Autodesk Inventor part; units mm, degrees
ref_plane "YZ Plane" through (0, 0, 0) normal (1, 0, 0) x (0, 1, 0)
ref_plane "XZ Plane" through (0, 0, 0) normal (0, 1, 0) x (-1, 0, 0)
ref_plane "XY Plane" through (0, 0, 0) normal (0, 0, 1) x (1, 0, 0)
sketch "Sketch1" plane through (0, 0, 0) normal (0, 0, 1) x (1, 0, 0)
  arc A0 (251, 0) -> (0, 251) centre (0, 0) ccw
  arc A1 (0, 355) -> (355, 0) centre (0, 0) ccw construction
  circle A2 centre (0, 0) radius 320 construction
  line L0 (0, 0) -> (0, 251) construction
  line L1 (0, 0) -> (251, 0) construction
  arc A3 (355, 0) -> (0, 355) centre (0, 0) ccw
  line L2 (0, 251) -> (0, 355)
  arc A4 (0, 251) -> (251, 0) centre (0, 0) ccw construction
  line L3 (251, 0) -> (355, 0)
  dimension "d0" = 502
  dimension "d1" = 710
  dimension "d2" = 640
extrude "Plate1" add sketch "Sketch1" against normal blind 4
sketch "Sketch3" plane through (0, 0, 0) normal (0, 0, 1) x (1, 0, 0)
  circle A0 centre (0, 0) radius 320 construction
  line L0 (0, 0) -> (0, 355) construction
  arc A1 (355, 0) -> (0, 355) centre (0, 0) ccw
  line L1 (0, 0) -> (55.5342, 350.6294) construction
  circle A2 centre (50.059, 316.0603) radius 16.5
  dimension "d12" = 640
  dimension "d13" = 9
  dimension "d14" = 33
extrude "Extrusion2" cut sketch "Sketch3" against normal through all
pattern_circular "Circular Pattern1" count 5 over 72 about axis through (0, 0, -10) along (0, 0, -1) of "Extrusion2"
equation "\"d5\" = Thickness"
equation "\"BendReliefWidth\" = Thickness"
equation "\"BendReliefDepth\" = 0.5 * Thickness"
equation "\"CornerReliefSize\" = 4 * Thickness"
equation "\"MinimumRemnant\" = 2 * Thickness"
equation "\"TransitionRadius\" = BendRadius"
equation "\"JacobiRadiusSize\" = BendRadius"
equation "\"GapSize\" = Thickness"
properties part number "MSC 036 flange 500" material "Stainless Steel"
Read the model definition and answer for the solid it produces. Units are mm, in the model's axes. Round coordinates to 2 decimals unless told otherwise and drop trailing zeros. Write each loop counter-clockwise with the first axis right and the second up, starting at its lowest first coordinate (ties: lowest second). Pieces come first, ordered by that corner, then holes.
1. The part is cut by section A-A, the plane x = 49.5. Determine the outline of the cut face in (y, z), then the cut area to 3 significant figures.
2. The part is cut by section B-B, the plane y = 44. Determine the outline of the cut face in (x, z), then the cut area to 3 significant figures.
3. Given pin 1 Ø20 at (x, y) = (50.06, 316.06) entering from +Z; pin 2 Ø2 at (x, z) = (153.5, -3.5) entering from +Y; pin 3 Ø1 at (x, z) = (156.5, -2) entering from -Y; pin 4 Ø1 at (x, z) = (55.5, -2) entering from +Y, each flat-ended and moving along its own axis, determine where each tip first touches the part or whether it passes through.
4. The part is cut by section D-D, the plane y = 260. Determine the outline of the cut face in (x, z), then the cut area to 3 significant figures.
5. Straight lines are drawn through the part: L1, parallel to X at y = 295, z = -0.45; L2, parallel to X at y = 39, z = -2.25 (3 decimals); L3, parallel to Y at x = 285.5, z = -0.6. For each, find the intervals that lie inside material, in ascending order.
6. Determine the mould class of faces 1 (the face through (179.425, 175.522, -1.972)), 2 (the face through (209.78, 225.85, -1.97)), 3 (the face through (253.768, 248.248, -1.972)), 4 (the face through (214, 180, -4)) for opening direction X: pulls with the +X half, pulls with the -X half, needs draft (parallel to the pull), parting line crosses it, or undercut.
Values:
1. outline: (246.07, -4) - (299.57, -4) - (299.57, 0) - (246.07, 0) - close; (332.55, -4) - (351.53, -4) - (351.53, 0) - (332.55, 0) - close
1. area: 290 mm2
2. outline: (247.11, -4) - (300.71, -4) - (300.71, 0) - (247.11, 0) - close; (331.41, -4) - (352.26, -4) - (352.26, 0) - (331.41, 0) - close
2. area: 298 mm2
3. pin 1: passes through
3. pin 2: stops at y = 320.58
3. pin 3: stops at y = 195.84
3. pin 4: stops at y = 350.71
4. outline: (0, -4) - (241.71, -4) - (241.71, 0) - (0, 0) - close
4. area: 967 mm2
5. L1: x = 0 to 132.06, 158.49 to 197.48
5. L2: x = 247.952 to 303.815, 328.306 to 352.851
5. L3: y = 0 to 128.78, 161.77 to 210.99
6. face 1: pulls with the -X half
6. face 2: undercut
6. face 3: pulls with the +X half
6. face 4: needs draft
